Autodesk Inventor part; units mm, degrees
ref_plane "YZ Plane" through (0, 0, 0) normal (1, 0, 0) x (0, 1, 0)
ref_plane "XZ Plane" through (0, 0, 0) normal (0, 1, 0) x (-1, 0, 0)
ref_plane "XY Plane" through (0, 0, 0) normal (0, 0, 1) x (1, 0, 0)
sketch "Sketch1" plane through (0, 0, 0) normal (1, 0, 0) x (0, 1, 0)
  line L0 (0, 0) -> (7.5, 0)
  line L1 (7.5, 0) -> (7.5, -20)
  line L2 (7.5, -20) -> (0, -20)
  line L3 (0, -20) -> (0, 0)
  circle A0 centre (3.75, -15.8984) radius 1.25
  dimension "d0" = 7.5
  dimension "d1" = 20
  dimension "d2" = 2.5
extrude "Extrusion1" add sketch "Sketch1" along normal blind 10
sketch "Sketch2" plane through (10, 0, 0) normal (1, 0, 0) x (0, 0, -1)
  line L0 (20, 7.5) -> (0, 7.5)
  line L1 (0, 7.5) -> (20, 7.5)
  line L2 (20, 7.5) -> (20, 0)
  line L3 (20, 0) -> (0, 0)
  line L4 (0, 0) -> (0, 7.5)
  circle A0 centre (15.8984, 3.75) radius 1.25
  circle A1 centre (15.8984, 3.75) radius 1.25
sketch "Sketch3" plane through (0, 7.5, 0) normal (0, 1, 0) x (1, 0, 0)
  point P0 (0, 0)
extrude "Extrusion2" add sketch "Sketch2" along normal blind 2 contours A0
sketch "Sketch4" plane through (10, 3.75, -15.8984) normal (-1, 0, 0) x (0, 0, 1)
  circle A0 centre (0, 0) radius 1.25
  point P0 (15.8984, -3.75)
extrude "Extrusion3" add sketch "Sketch4" along normal blind 10
properties part number "servo"
The listing builds one solid part. Answer for the finished solid, in the listing's coordinates (mm). A direction names the side the tool comes from. Give positions to 0.01 mm unless a question says otherwise; leave off trailing zeros. Write each loop counter-clockwise with the first axis right and the second up, starting at its lowest first coordinate (ties: lowest second). Pieces come first, ordered by that corner, then holes.
Item 1: Section C-C, the plane y = 2 is taken. Write down the section's boundary in (x, z).
Item 2: Section B-B, the plane z = -16.5 is taken. Write down the section's boundary in (x, y).
Item 3: Section A-A, the plane y = 3.75 is taken. Write down the section's boundary in (x, z), plus the area to 3 significant figures.
Item 4: Section D-D, the plane z = -13.5 is taken. Write down the section's boundary in (x, y).
Item 5: Flat-ended cylindrical pins translate along their axes: P1, Ø5, axis at x = 3.5, z = -14.5, coming from the -Y side; P2, Ø1.5, axis at y = 3, z = -12, coming from the +X side. Find the tip coordinate at first contact, or state that the pin passes through.
Item 6: Find the intervals of material crossed by line 1 along X through (y, z) = (0.5, -1), in increasing order.
Item 7: Which of the six approach directions +Z, -Z, +X, -X, +Y, -Y give full straight-line access (tool end or side, diameter ignored) to faces 1 (the flat face through (5, 7.5, -10)), 2 (the cylindrical face through (10.99, 4.97, -15.63))?
Completed:
1. outline: (0, -20) - (10, -20) - (10, 0) - (0, 0) - close
2. outline: (0, 0) - (10, 0) - (10, 2.65) - (12, 2.65) - (12, 4.85) - (10, 4.85) - (10, 7.5) - (0, 7.5) - close
3. outline: (0, -20) - (10, -20) - (10, -17.15) - (12, -17.15) - (12, -14.65) - (10, -14.65) - (10, 0) - (0, 0) - close
3. area: 205 mm2
4. outline: (0, 0) - (10, 0) - (10, 7.5) - (0, 7.5) - close
5. P1: stops at y = 0
5. P2: stops at x = 10
6. line 1: x = 0 to 10
7. face 1: +Z, -Z, +X, -X, +Y
7. face 2: +X
